from build123d import *

# Parameters (mm, degrees)
F0_R            = 300
F1_DEPTH        = 48
F2_R            = 235
F3_DEPTH        = 5
F5_D            = 17.5
F5_COPIES_COUNT = 16
F6_R            = 205
F7_DEPTH        = 53.001
F9_D            = 22
F9_START        = 5
F9_CBORE_D      = 32
F9_CBORE_DEPTH  = 30
F9_COPIES_COUNT = 24


# Not quite as in the source:
# - a pattern or mirror of a feature is missing from the dataset's text; its kind, count and spacing are read off the source's solid


with BuildPart() as f1:
    # F0 (on Front) → F1 (new body)
    with BuildSketch(Plane.XZ):
        Circle(F0_R)
    extrude(amount=F1_DEPTH)

    # F2 (on face) → F3 (join)
    with BuildSketch(Plane.XZ.offset(48)):
        Circle(F2_R)
    extrude(amount=F3_DEPTH)

    # F5 (through all)
    with Locations(Plane.XZ.offset(48)):
        with Locations((0, 280)):
            f5 = Hole(F5_D / 2)

    # F5_copies: F5 ×16 about axis
    f5_copies_axis = Axis((0, 0, 0), (0, 1, 0))
    for i in range(1, F5_COPIES_COUNT):
        add(f5.rotate(f5_copies_axis, i * 360 / F5_COPIES_COUNT), mode=Mode.SUBTRACT)

    # F6 (on face) → F7 (cut, through all)
    with BuildSketch(Plane(origin=(0, 0, 0), x_dir=(-1, 0, 0), z_dir=(0, 1, 0))):
        Circle(F6_R)
    extrude(amount=-F7_DEPTH, mode=Mode.SUBTRACT)

    # F9 (through all)
    # its depths count from where the whole tool has entered the part; down to there all is cleared
    with Locations(Plane.XZ.offset(53).offset(-F9_START)):
        with Locations((0, 230)):
            f9 = CounterBoreHole(F9_D / 2, F9_CBORE_D / 2, F9_CBORE_DEPTH)

    # F9_copies: F9 ×24 about axis
    f9_copies_axis = Axis((0, 0, 0), (0, 1, 0))
    for i in range(1, F9_COPIES_COUNT):
        add(f9.rotate(f9_copies_axis, i * 360 / F9_COPIES_COUNT), mode=Mode.SUBTRACT)

    # F9_copies1: F9 across plane
    add(f9.mirror(Plane(origin=(0, 0, 0), x_dir=(-0.9914448614, 0, 0.1305261922), z_dir=(-0.1305261922, 0, -0.9914448614))), mode=Mode.SUBTRACT)


solid = f1.part
The listing builds one solid part. Answer for the finished solid, in the listing's coordinates (mm). A direction names the side the tool comes from. Give positions to 0.01 mm unless a question says otherwise; leave off trailing zeros. Loops run counter-clockwise (first coordinate to the right, second up) from the corner with the lowest first, then second, coordinate; pieces in that order, holes last. Notation, with made-up numbers: (65.5, 18) - (95.5, 18) arc R10 cw to (95.5, 24) - close; hole circle Ø8 at (-0.75, 19.5). An arc over 180 degrees is marked (long way). Write each question's results on one line, items separated by ' | '.
1. Find section C-C, the plane x = 163. Write down the section's boundary in (y, z).
Resolved:
outline: (-53, -146.64) - (-18, -146.64) - (-18, -151.64) - (0, -151.64) - (0, -124.32) - (-53, -124.32) - close; (-53, 124.32) - (0, 124.32) - (0, 151.64) - (-18, 151.64) - (-18, 146.64) - (-53, 146.64) - close; (-48, -251.86) - (0, -251.86) - (0, -173.63) - (-18, -173.63) - (-18, -178.63) - (-48, -178.63) - close; (-48, 178.63) - (-18, 178.63) - (-18, 173.63) - (0, 173.63) - (0, 251.86) - (-48, 251.86) - close
2. Flat-ended cylindrical pins translate along their axes: P1, Ø6, axis at x = -43, y = -6.5, coming from the -Z side; P2, Ø9.5, axis at x = -216.5, z = -54.5, coming from the -Y side; P3, Ø8, axis at x = -81, y = -29, coming from the +Z side. Find the tip coordinate at first contact, or state that the pin passes through.
Resolved:
P1: stops at z = -297.32 | P2: stops at y = -18 | P3: stops at z = 289.95
3. Find section D-D, the plane x = 280. Write down the section's boundary in (y, z).
Resolved:
outline: (-48, -107.7) - (0, -107.7) - (0, -8.75) - (-48, -8.75) - close; (-48, 8.75) - (0, 8.75) - (0, 107.7) - (-48, 107.7) - close
4. Find section A-A, the plane x = 0. Count the separate pieces of the cut face and the enclosed holes in it, then the cut area to 3 significant figures.
Resolved:
separate pieces: 6 | enclosed holes: 0 | area: 4,820 mm^2
5. Which of the six approach directions +Z, -Z, +X, -X, +Y, -Y give full straight-line access (tool end or side, diameter ignored) to faces 5 (the face through (155.21, -8.87, -170.75)), 6 (the face through (-197, -18, 126))?
Resolved:
face 5: +Y, -Y | face 6: -Y
6. Consider probe 1 along Z at (x, y) = (266, -39.5); probe 2 along Z at (x, y) = (-221, -3); probe 3 along X at (y, z) = (-41, -115). Determine where each line is inside the solid, lowest interval first. Write a range as from..to.
Resolved:
probe 1: z = -138.72..-111.95, -102.35..102.35, 111.95..138.72 | probe 2: z = -202.88..-70.47, -48.59..-6.32, 6.32..48.59, 70.47..202.88 | probe 3: x = -277.08..-262.55, -254.82..-215.19, -183.19..-169.71, 169.71..183.19, 215.19..254.82, 262.55..277.08
7. For a pull along Z with two mould halves and no side action, classify faces 1 (the face through (62, 0, -196)), 2 (the face through (186.57, -50.46, 142.89)), 3 (the face through (188, -18, 113)), 4 (the face through (-143.23, -50.465, -186.307)) as +Z half, -Z half, draft (parallel to the pull), parting line (faces both ways), or undercut.
Resolved:
face 1: draft | face 2: +Z half | face 3: undercut | face 4: -Z half
8. Find section B-B, the plane z = -280. Write down the section's boundary in (x, y).
Resolved:
outline: (-107.7, -48) - (-8.75, -48) - (-8.75, 0) - (-107.7, 0) - close; (8.75, -48) - (107.7, -48) - (107.7, 0) - (8.75, 0) - close
